from build123d import *

# Parameters (mm, degrees)
SKETCH1_R                      = 4.95
SKETCH1_W                      = 17.9
SKETCH1_H                      = 45.1
BOSS_EXTRUDE1_DEPTH            = 3
CUT_EXTRUDE1_DEPTH             = 251.790202921
CUT_EXTRUDE1_DEPTH_BACK        = 251.790202921
SKETCH2_W                      = 258.160615752
SKETCH2_H                      = 10
SKETCH3_W                      = 12
SKETCH3_H                      = 60
BOSS_EXTRUDE2_DEPTH            = 3
FILLET1_R                      = 20
BOSS_EXTRUDE3_START            = -3
BOSS_EXTRUDE3_DEPTH            = 3
CIRPATTERN1_COUNT              = 9
SKETCH5_W                      = 17
SKETCH5_H                      = 3.1
CUT_EXTRUDE2_DEPTH             = 250.90439271
CUT_EXTRUDE3_DEPTH             = 250.90439271
MAIN_SHAFT_CLEARANCE_PROFILE_R = 5.05
SHAFT_CLEARANCE_10P1_DEPTH     = 250.90439271


with BuildPart() as part:
    # Sketch1 → Boss-Extrude1 (new body)
    with BuildSketch(Plane.YZ):
        with BuildLine():
            Line((-10.899695646, -10.305175148), (-129.080307876, -215))
            Line((-129.080307876, -215), (-88.665789032, -215))
            Line((-88.665789032, -215), (-17.790269987, -92.24))
            Line((-17.790269987, -92.24), (17.790269987, -92.24))
            Line((17.790269987, -92.24), (88.665789032, -215))
            Line((88.665789032, -215), (129.080307876, -215))
            Line((129.080307876, -215), (10.899695646, -10.305175148))
            ThreePointArc((10.899695646, -10.305175148), (0, 15), (-10.899695646, -10.305175148))
        make_face()
        with Locations(Location((0, 0, 0), (0, 0, 270))):
            Circle(SKETCH1_R, mode=Mode.SUBTRACT)
        with Locations((0, -54.69)):
            Rectangle(SKETCH1_W, SKETCH1_H, mode=Mode.SUBTRACT)
    extrude(amount=BOSS_EXTRUDE1_DEPTH)

    # Sketch2 → Cut-Extrude1 (cut, two sides: drawn at the far end of the back side and taken through both)
    with BuildSketch(Plane.YZ.offset(3).offset(-CUT_EXTRUDE1_DEPTH_BACK)):
        with Locations((0, -210)):
            Rectangle(SKETCH2_W, SKETCH2_H)
    extrude(amount=CUT_EXTRUDE1_DEPTH + CUT_EXTRUDE1_DEPTH_BACK, mode=Mode.SUBTRACT)

    # Sketch3 → Boss-Extrude2 (add)
    with BuildSketch(Plane(origin=(3, 0, 0), x_dir=(0, 0, -1), z_dir=(1, 0, 0))):
        with Locations((199, -112.892286341)):
            Rectangle(SKETCH3_W, SKETCH3_H)
        with Locations((199, 112.892286341)):
            Rectangle(SKETCH3_W, SKETCH3_H)
    extrude(amount=-BOSS_EXTRUDE2_DEPTH)

    # Fillet1
    fillet1_edges = [part.edges().sort_by_distance(p)[0] for p in [
        (1.5, -116.378601954, -193),
        (1.5, 116.378601954, -193),
    ]]
    fillet(fillet1_edges, radius=FILLET1_R)

    # Sketch4 → Boss-Extrude3 (add)
    with BuildSketch(Plane(origin=(3, 0, 0), x_dir=(0, 0, -1), z_dir=(1, 0, 0)).offset(BOSS_EXTRUDE3_START)):
        with BuildLine():
            Line((-14.095389312, 5.13030215), (-34.137962787, 0))
            Line((-34.137962787, 0), (-15, 0))
            ThreePointArc((-15, 0), (-14.772116295, 2.604722665), (-14.095389312, 5.13030215))
        make_face()
        with BuildLine():
            Line((-34.137962787, 0), (-14.095389312, -5.13030215))
            ThreePointArc((-14.095389312, -5.13030215), (-14.772116295, -2.604722665), (-15, 0))
            Line((-15, 0), (-34.137962787, 0))
        make_face()
    boss_extrude3 = extrude(amount=BOSS_EXTRUDE3_DEPTH)

    # CirPattern1: Boss-Extrude3 ×9 about axis
    cirpattern1_axis = Axis((0, 0, 0), (1, 0, 0))
    for i in range(1, CIRPATTERN1_COUNT):
        add(boss_extrude3.rotate(cirpattern1_axis, i * 360 / CIRPATTERN1_COUNT))

    # Sketch5 → Cut-Extrude2 (cut, symmetric)
    with BuildSketch(Plane(origin=(3, 0, 0), x_dir=(0, 0, -1), z_dir=(1, 0, 0))):
        with Locations((191.5, -126.342286341)):
            Rectangle(SKETCH5_W, SKETCH5_H)
    cut_extrude2 = extrude(amount=CUT_EXTRUDE2_DEPTH, both=True, mode=Mode.SUBTRACT)

    # Mirror1: Cut-Extrude2 across plane
    add(cut_extrude2.mirror(Plane.ZX), mode=Mode.SUBTRACT)

    # Sketch6 → Cut-Extrude3 (cut, symmetric)
    with BuildSketch(Plane.YZ.offset(3)):
        Polygon((-15.413378072, -72.19421526), (-14.95, -71.844331927), (-14.95, -32.59506202), (-19.146348264, -44.729209649), (-33.320603167, -85.715441185), (-16.757760632, -73.209319511), align=None)
        Polygon((-40.452020015, -87.978847078), (-27.957868434, -51.850797102), (-58.475794969, -104.709396402), (-41.912952433, -92.203274728), align=None)
        Polygon((-44.440620352, -126.565865893), (-18.81339339, -82.279763058), (-34.966746745, -94.476691336), (-36.374058239, -98.54606889), align=None)
        Polygon((-53.243788825, -135.456403713), (-43.245914121, -100.728050325), (-59.700544534, -113.152464165), (-68.824966717, -146.420983438), align=None)
        Polygon((-80.442842118, -188.780872527), (-54.234238638, -143.490099921), (-68.345208144, -153.420084111), (-71.318419935, -155.512353255), align=None)
        Polygon((-76.978433226, -153.464848336), (-68.249306861, -121.637615567), (-99.099637478, -175.071955626), (-80.672732205, -157.159147315), align=None)
        Polygon((-112.914500338, -199), (-89.467175046, -199), (-88.913955872, -196.982909779), (-80.146284863, -165.015139537), (-102.228944471, -186.481709354), (-110.110561046, -194.143434684), align=None)
    cut_extrude3 = extrude(amount=CUT_EXTRUDE3_DEPTH, both=True, mode=Mode.SUBTRACT)

    # Mirror2: Cut-Extrude3 across plane
    add(cut_extrude3.mirror(Plane.ZX), mode=Mode.SUBTRACT)

    # Main_shaft_clearance_profile → Shaft_clearance_10p1 (cut, through all)
    with BuildSketch(Plane.YZ):
        with Locations(Location((0, 0, 0), (0, 0, 90))):
            Circle(MAIN_SHAFT_CLEARANCE_PROFILE_R)
    extrude(amount=SHAFT_CLEARANCE_10P1_DEPTH, mode=Mode.SUBTRACT)


solid = part.part
Here's how the part is built. I have some questions about the finished solid (model axes, mm). A direction names the side the tool comes from. Coordinates: 2 decimals unless noted, no trailing zeros.
1) If I drill on line 1 (Y direction, x = 0.25, z = -71.5); line 2 (Y direction, x = 0.2, z = -93); line 3 (Y direction, x = 0.35, z = -43), over which ranges is the centre line in solid material (lowest first)?
Filled in:
line 1: y = -46.23 to -39.3, -34.75 to -28.4, -14.95 to -8.95, 8.95 to 14.95, 28.4 to 34.75, 39.3 to 46.23
line 2: y = -58.64 to -51.72, -42.97 to -33.01, -25.02 to -18.23, 18.23 to 25.02, 33.01 to 42.97, 51.72 to 58.64
line 3: y = -29.78 to -18.55, -14.95 to -8.95, 8.95 to 14.95, 18.55 to 29.78
2) I'm going to push flat-ended pins straight in: pin 1 (1.5 mm diameter, centred on x = 1.5, z = -115, fed in from -Y); pin 2 (0.9 mm diameter, centred on x = 2, z = -44.5, fed in from -Y); pin 3 (0.9 mm diameter, centred on x = 2, y = -106.5, fed in from +Z); pin 4 (9 mm diameter, centred on y = 0, z = 0, fed in from -X). Where does each tip first touch, or does it pass through?
Filled in:
pin 1: stops at y = -71.78
pin 2: stops at y = -30.9
pin 3: stops at z = -175.11
pin 4: passes through
3) If we section it at A-A (x = 2.1): Count the separate pieces of the cut face and the enclosed holes in it, plus the area to 3 significant figures.
Filled in:
separate pieces: 1
enclosed holes: 16
area: 11,400 mm2
4) Thinking about a two-plate mould opening in Y: for faces 1 (the face through (3, -7, -92)), 2 (the face through (1.479, -26.777, -88.293)), 3 (the face through (1.48, 24.06, 1.6)), which applies, +Y half, -Y half, draft (parallel to the pull), parting line (faces both ways), or undercut?
Filled in:
face 1: draft
face 2: undercut
face 3: +Y half
5) Which directions (+Z, -Z, +X, -X, +Y, -Y) give clear straight access to the entire face, cutting with the end or side of a thin tool? Please do faces 4 (the face through (1.479, 49.886, -147.831)), 5 (the face through (1.479, -22.065, -9.736)), 6 (the face through (1.521, 116.698, -189.551)).
Filled in:
face 4: -Z, +X, -X
face 5: +X, -X, -Y
face 6: +Z, +X, -X, +Y
